Source: CAD feature listing. Evaluate the final solid. Frame: model axes, mm. Face numbers are marked on the shaded views. A direction names the side the tool comes from. Coordinates: 2 decimals unless noted, no trailing zeros. Loops run counter-clockwise (first coordinate to the right, second up) from the corner with the lowest first, then second, coordinate; pieces in that order, holes last.
Autodesk Inventor part; units mm, degrees
ref_plane "YZ Plane" through (0, 0, 0) normal (1, 0, 0) x (0, 1, 0)
ref_plane "XZ Plane" through (0, 0, 0) normal (0, 1, 0) x (-1, 0, 0)
ref_plane "XY Plane" through (0, 0, 0) normal (0, 0, 1) x (1, 0, 0)
sketch "Sketch2" plane through (0, 0, 0) normal (0, 1, 0) x (-1, 0, 0)
  line L0 (-2.75, -2.75) -> (2.75, -2.75)
  line L1 (2.75, -2.75) -> (2.75, 2.75)
  line L2 (2.75, 2.75) -> (-2.75, 2.75)
  line L3 (-2.75, 2.75) -> (-2.75, -2.75)
  line L4 (-2.75, -2.75) -> (2.75, 2.75) construction
  line L5 (2.75, -2.75) -> (-2.75, 2.75) construction
  line L6 (3.25, 3.25) -> (-3.25, 3.25)
  line L7 (-3.25, 3.25) -> (-3.25, -3.25)
  line L8 (-3.25, -3.25) -> (3.25, -3.25)
  line L9 (3.25, -3.25) -> (3.25, 3.25)
  line L10 (3.25, 3.25) -> (-3.25, -3.25) construction
  line L11 (-3.25, 3.25) -> (3.25, -3.25) construction
  point P0 (0, 0)
  dimension "d2" = 5.5
  dimension "d3" = 5.5
  dimension "d6" = 6.5
  dimension "d7" = 6.5
extrude "Extrusion1" add sketch "Sketch2" along normal blind 2
sketch "Sketch4" plane through (0, 2, 0) normal (0, 1, 0) x (1, 0, 0)
  line L0 (-3.25, 3.25) -> (-3.25, -3.25)
  line L1 (3.25, -3.25) -> (3.25, 3.25)
  line L2 (-3.25, -3.25) -> (3.25, -3.25)
  line L3 (3.25, -3.25) -> (3.25, 3.25)
  line L4 (3.25, 3.25) -> (-3.25, 3.25)
  line L5 (-3.25, 3.25) -> (-3.25, -3.25)
  point P0 (0, 0)
  dimension "d10" = 6.5
extrude "Extrusion2" add sketch "Sketch4" along normal blind 1
properties part number "snapfit_lid_v03"
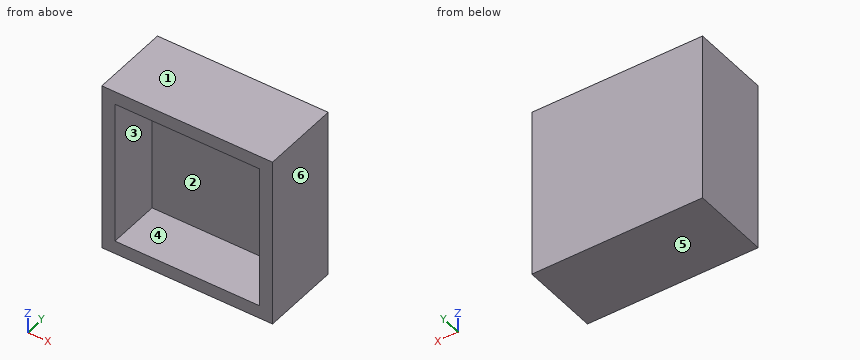
Q1. First-contact query: pin 1 Ø2 at (x, z) = (-1, -1.5) entering from -Y. Flat tip, straight axial feed; report the tip coordinate or a pass-through.
Q2. Section query B-B on z = -1. Return the cut outline in (x, y).
Q3. Section query C-C on x = 1. Return the cut outline in (y, z), then the cut area to 3 significant figures.
Q4. Draft query along Z for the marked faces 3, 4, 5 and 6. Return one class per face: released by +Z, released by -Z, zero draft, split by the parting line, or undercut.
Q5. Material intervals for line 1 along X through (y, z) = (0.2, 1.25); line 2 along Y through (x, z) = (-0.5, 0), sorted ascending.
Q6. Section query A-A on y = 1. Return the cut outline in (x, z), then the cut area to 3 significant figures.
Q7. Reachability of the marked faces 1 and 2 from +Z, -Z, +X, -X, +Y, -Y: full face, straight path, thin tool, end or side. Return the list, or none.
Resolved:
1. pin 1: stops at y = 2
2. outline: (-3.25, 0) - (-2.75, 0) - (-2.75, 2) - (2.75, 2) - (2.75, 0) - (3.25, 0) - (3.25, 3) - (-3.25, 3) - close
3. outline: (0, -3.25) - (3, -3.25) - (3, 3.25) - (0, 3.25) - (0, 2.75) - (2, 2.75) - (2, -2.75) - (0, -2.75) - close
3. area: 8.50 mm2
4. face 3: undercut
4. face 4: undercut
4. face 5: released by -Z
4. face 6: zero draft
5. line 1: x = -3.25 to -2.75, 2.75 to 3.25
5. line 2: y = 2 to 3
6. outline: (-3.25, -3.25) - (3.25, -3.25) - (3.25, 3.25) - (-3.25, 3.25) - close; hole (-2.75, -2.75) - (2.75, -2.75) - (2.75, 2.75) - (-2.75, 2.75) - close
6. area: 12.0 mm2
7. face 1: +Z, +X, -X, +Y, -Y
7. face 2: -Y
